Autodesk Fusion 360 part; units mm, degrees
sketch "Sketch1" plane through (0, 0, 0) normal (0, 0, 1) x (1, 0, 0)
  line L0 (0, 0) -> (40, 0)
  line L1 (40, 0) -> (40, 20)
  line L2 (40, 20) -> (0, 20)
  line L3 (0, 20) -> (0, 0)
  dimension "d1" = 40
  dimension "d2" = 20
extrude "Extrude1" add sketch "Sketch1" along normal blind 20
sketch "Sketch2" plane through (0, 0, 0) normal (0, 0, -1) x (1, 0, 0)
  line L0 (0, 0) -> (0, -20)
  line L1 (0, -20) -> (40, -20)
  line L2 (40, -20) -> (40, 0)
  line L3 (40, 0) -> (0, 0)
  line L4 (0, 0) -> (10, 0)
  line L5 (10, 0) -> (10, -20)
  line L6 (10, -20) -> (0, -20)
  line L7 (0, -20) -> (0, 0)
  line L8 (10, -10) -> (23.8, -10)
  circle A0 centre (23.8, -10) radius 3.25
  dimension "d5" = 10
  dimension "d6" = 20
  dimension "d7" = 13.8
  dimension "d8" = 6.5
extrude "Extrude2" cut sketch "Sketch2" against normal blind 7.8 contours L0 L1 L3 L4 L5 L6 L7 | A0
extrude "Extrude3" cut 1 faces at (24.5115, 8.6722, 7.8) along direction (0, 0, 1) blind 210
sketch "Sketch3" plane through (0, 0, 20) normal (0, 0, 1) x (-1, 0, 0)
  circle A0 centre (-23.8, -10) radius 3.25
  line L0 (0, -20) -> (0, 0)
  line L1 (0, 0) -> (-40, 0)
  line L2 (-40, 0) -> (-40, -20)
  line L3 (-40, -20) -> (0, -20)
  line L4 (-40, -20) -> (-15, -20)
  line L5 (-15, -20) -> (-15, 0)
  line L6 (-15, 0) -> (-40, 0)
  line L7 (-40, 0) -> (-40, -20)
  dimension "d13" = 25
  dimension "d14" = 20
extrude "Extrude4" cut sketch "Sketch3" against normal blind 10 contours L1 L2 L3 L4 L5 L6 L7
fillet "Fillet1" radius 5 2 edges at (15, 10, 10) (15, 10, 20)
fillet "Fillet2" radius 5 2 edges at (40, 0, 5) (40, 20, 5)
sketch "Sketch4" plane through (0, 0, 0) normal (0, 1, 0) x (1, 0, 0)
extrude "Extrude5" cut 1 faces at (10, 6.6667, 2.6) along direction (1, 0, 0) blind 0.5
extrude "Extrude6" add 1 faces at (10.5, 6.6667, 2.6) along direction (-1, 0, 0) blind 0.5
sketch "Sketch5" plane through (0, 0, 20) normal (0, 0, 1) x (-1, 0, 0)
  line L0 (-10, 0) -> (-10, -20)
  line L1 (-10, -20) -> (0, -20)
  line L2 (0, -20) -> (0, 0)
  line L3 (0, 0) -> (-10, 0)
sketch "Sketch6" plane through (0, 0, 0) normal (0, -1, 0) x (1, 0, 0)
  line L0 (10, 0) -> (35, 0)
  line L1 (35, 0) -> (35, 10)
  line L2 (35, 10) -> (20, 10)
  arc A0 (15, 15) -> (20, 10) centre (20, 15) ccw
  arc A1 (15, 15) -> (10, 20) centre (10, 15) ccw
  line L3 (10, 20) -> (0, 20)
  line L4 (0, 20) -> (0, 7.8)
  line L5 (0, 7.8) -> (10, 7.8)
  line L6 (10, 7.8) -> (10, 0)
sketch "Sketch7" plane through (0, 0, 0) normal (0, -1, 0) x (1, 0, 0)
sketch "Sketch8" plane through (0, 0, 10) normal (0, 0, 1) x (-1, 0, 0)
  arc A0 (-40, -15) -> (-35, -20) centre (-35, -15) ccw
  line L0 (-35, -20) -> (-20, -20)
  line L1 (-20, -20) -> (-20, 0)
  line L2 (-20, 0) -> (-35, 0)
  arc A1 (-35, 0) -> (-40, -5) centre (-35, -5) ccw
  line L3 (-40, -5) -> (-40, -15)
  circle A2 centre (-23.8, -10) radius 3.25
extrude "Extrude7" add 1 faces at (3.3333, 6.6667, 7.8) along direction (0, 0, -1) blind 1
For this review, take the finished solid that the model builds, in its own axes (mm). A direction names the side the tool comes from. Coordinates: 2 decimals unless noted, no trailing zeros. Loops run counter-clockwise (first coordinate to the right, second up) from the corner with the lowest first, then second, coordinate; pieces in that order, holes last. Notation, with made-up numbers: (6.5, 39.5) - (22.5, 39.5) arc R18 ccw to (22.5, 47.5) - close; hole circle Ø7 at (-4, -0.75). An arc over 180 degrees is marked (long way). Return JSON: item names as keys, results as strings.
Item 1: Mouldability with a two-part tool opening along Y and no side actions: class faces 1 (the cylindrical face through (38, 1, 5)), 2 (the cylindrical face through (20.553, 9.857, 4.93)), 3 (the flat face through (17, 20, 8)), 4 (the cylindrical face through (16, 10, 12)) as pulls with the +Y half, pulls with the -Y half, needs draft (parallel to the pull), parting line crosses it, or undercut.
Determined:
{"face 1": "pulls with the -Y half", "face 2": "undercut", "face 3": "pulls with the +Y half", "face 4": "needs draft"}
Item 2: Insertion check: pin 1 (6 mm diameter, centred on x = 33.5, y = 12.5, fed in from +Z); pin 2 (4 mm diameter, centred on y = 17.5, z = 9.5, fed in from +X); pin 3 (2 mm diameter, centred on y = 8, z = 4.5, fed in from -X). Each pin has a flat end and moves straight along its axis. Give the tip position at first contact, or say it passes through.
Determined:
{"pin 1": "stops at z = 10", "pin 2": "stops at x = 39.97", "pin 3": "stops at x = 10"}
Item 3: For line 1 (Y direction, x = 23.8, z = 5.75); line 2 (X direction, y = 10, z = 7); line 3 (X direction, y = 10, z = 6.5), list the stretches that pass through material, from the lowest coordinate up.
Determined:
{"line 1": "y = 0 to 6.75, 13.25 to 20", "line 2": "x = 0 to 20.55, 27.05 to 40", "line 3": "x = 10 to 20.55, 27.05 to 40"}
Item 4: Take a section at B-B (z = 8). Give the boundary of the cut face in (x, y), then the cut area to 3 significant figures.
Determined:
{"outline": "(0, 0) - (35, 0) arc R5 ccw to (40, 5) - (40, 15) arc R5 ccw to (35, 20) - (0, 20) - close; hole circle Ø6.5 at (23.8, 10)", "area": "756 mm2"}
Item 5: For faces 5 (the flat face through (10, 10, 3)), 6 (the cylindrical face through (39, 18, 5)), 7 (the flat face through (30, 10, 10)), list the 3-axis set-ups (+Z, -Z, +X, -X, +Y, -Y) from which the entire face can be reached by the end or side of a thin tool; tool diameter is ignored.
Determined:
{"face 5": "-Z, -X, +Y, -Y", "face 6": "+Z, -Z, +X, +Y", "face 7": "+Z, +X, +Y, -Y"}
Item 6: Take a section at C-C (x = 23.8). Give the boundary of the cut face in (y, z).
Determined:
{"outline": "(0, 0) - (6.75, 0) - (6.75, 10) - (0, 10) - close; (13.25, 0) - (20, 0) - (20, 10) - (13.25, 10) - close"}
